The listing builds one solid part. Answer for the finished solid, in the listing's coordinates (mm). Give positions to 0.01 mm unless a question says otherwise; leave off trailing zeros. Order: outer loops, then holes, each group sorted by start corner. A loop starts at its lowest first (then second) coordinate and runs counter-clockwise, first axis right, second up. Notation, with made-up numbers: (-23, 79.25) - (-19, 79.25) arc R12 cw to (-19, 92.25) - close; hole circle Ø1 at (51.25, -30). An arc over 180 degrees is marked (long way). Answer as CSV lines item,"result". Start each with the question number.
1. Section C-C on z = 0.65 is taken. Count the separate pieces of the cut face and the enclosed holes in it, and give its area (3 significant figures).
2. A flat-ended cylindrical pin translates along its axis: pin 1 (1 mm diameter, centred on x = 4, z = 1.5, fed in from +Y). Find the tip coordinate at first contact, or state that the pin passes through.
3. Section B-B on y = -9 is taken. Give the vertices of the cut face in (x, z), and give its area (3 significant figures).
4. Section A-A on y = 1 is taken. Give the vertices of the cut face in (x, z).
5. Consider line 1 along X through (y, z) = (0.5, 1.5); line 2 along X through (y, z) = (-10.5, 0.4); line 3 along Y through (x, z) = (12.25, 0.45). Determine where each line is inside the solid, lowest interval first. Write a range as [from, to].
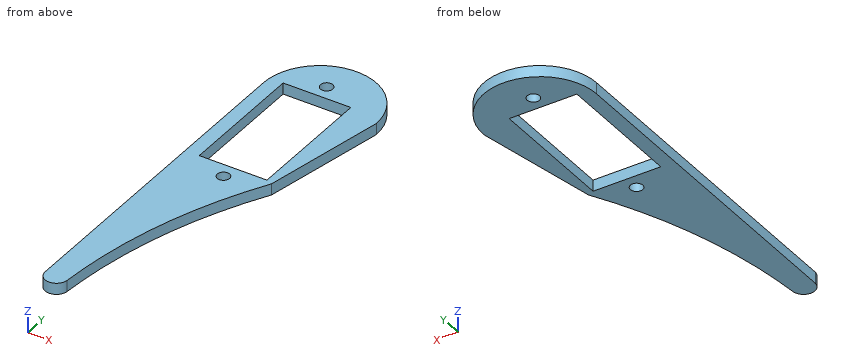
from build123d import *

# Parameters (mm, degrees)
BOSS_EXTRUDE1_DEPTH = 2
CUT_EXTRUDE1_REACH  = 64.284
SKETCH2_R           = 1.1
SKETCH2_W           = 12
SKETCH2_H           = 23


with BuildPart() as part:
    # Sketch1 → Boss-Extrude1 (new body)
    with BuildSketch(Plane.XY):
        with BuildLine():
            Line((-1.783693844, 2.329450915), (-1.783693844, -57.670549085))
            ThreePointArc((-1.783693844, -57.670549085), (0.216306156, -59.527300355), (2.216306156, -57.670549085))
            add(Edge.make_bspline(
                [(13.829397999, -19.605089871), (7.097626367, -31.400579811), (3.226595753, -44.089066216), (2.216306156, -57.670549085)],
                knots=[0, 0, 0, 0, 1, 1, 1, 1], degree=3))
            Line((13.829397999, -19.605089871), (18.216306156, 2.329450915))
            ThreePointArc((18.216306156, 2.329450915), (8.216306156, 12.329450915), (-1.783693844, 2.329450915))
        make_face()
    extrude(amount=BOSS_EXTRUDE1_DEPTH)

    # Sketch2 → Cut-Extrude1 (cut, up to next)
    with BuildSketch(Plane.XY.offset(2), mode=Mode.PRIVATE) as cut_extrude1_sk1:
        with Locations((6.716306156, 6.510600008)):
            Circle(SKETCH2_R)
    cut_extrude1_tool1 = extrude(cut_extrude1_sk1.sketch, amount=-CUT_EXTRUDE1_REACH, mode=Mode.PRIVATE) & part.part
    # Sketch2 → Cut-Extrude1 (cut, up to next)
    with BuildSketch(Plane.XY.offset(2), mode=Mode.PRIVATE) as cut_extrude1_sk2:
        with Locations((6.716306156, -21.789399992)):
            Circle(SKETCH2_R)
    cut_extrude1_tool2 = extrude(cut_extrude1_sk2.sketch, amount=-CUT_EXTRUDE1_REACH, mode=Mode.PRIVATE) & part.part
    # Sketch2 → Cut-Extrude1 (cut, up to next)
    with BuildSketch(Plane.XY.offset(2), mode=Mode.PRIVATE) as cut_extrude1_sk3:
        with Locations((6.716306156, -7.639399992)):
            Rectangle(SKETCH2_W, SKETCH2_H)
    cut_extrude1_tool3 = extrude(cut_extrude1_sk3.sketch, amount=-CUT_EXTRUDE1_REACH, mode=Mode.PRIVATE) & part.part
    add(cut_extrude1_tool1.solids().sort_by_distance((6.716306, 6.5106, 2))[0], mode=Mode.SUBTRACT)
    add(cut_extrude1_tool2.solids().sort_by_distance((6.716306, -21.7894, 2))[0], mode=Mode.SUBTRACT)
    add(cut_extrude1_tool3.solids().sort_by_distance((6.716306, -7.6394, 2))[0], mode=Mode.SUBTRACT)


solid = part.part
Checks:
1,separate pieces,"1"
1,enclosed holes,"3"
1,area,"583 mm²"
2,pin 1,"stops at y = 11.61"
3,outline,"(-1.78, 0) - (0.72, 0) - (0.72, 2) - (-1.78, 2) - close; (12.72, 0) - (15.95, 0) - (15.95, 2) - (12.72, 2) - close"
3,area,"11.5 mm²"
4,outline,"(-1.78, 0) - (0.72, 0) - (0.72, 2) - (-1.78, 2) - close; (12.72, 0) - (17.95, 0) - (17.95, 2) - (12.72, 2) - close"
5,line 1,"x = [-1.78, 0.72], [12.72, 17.85]"
5,line 2,"x = [-1.78, 0.72], [12.72, 15.65]"
5,line 3,"y = [-22.49, -19.14], [3.86, 11.48]"
